Check sheet for the modelled part. Datum: model origin and axes. Units: mm. Face numbers are marked on the shaded views. A direction names the side the tool comes from. Give positions to 0.01 mm unless a question says otherwise; leave off trailing zeros. Order: outer loops, then holes, each group sorted by start corner. A loop starts at its lowest first (then second) coordinate and runs counter-clockwise, first axis right, second up.
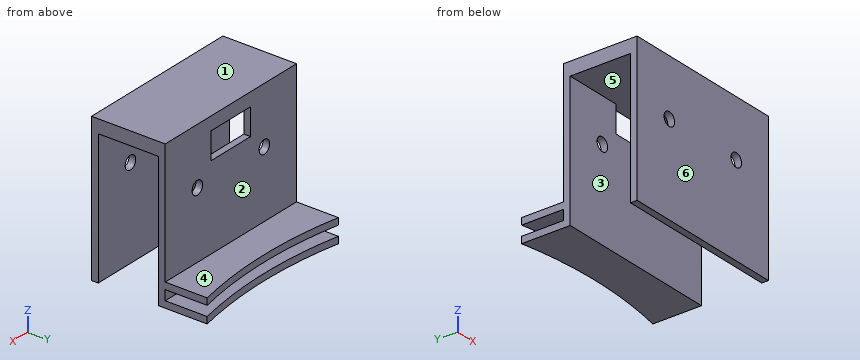
```python
from build123d import *

# Parameters (mm, degrees)
SKETCH_1_W          = 50
SKETCH_1_H          = 44
EXTRUDE_1_DEPTH     = 22
SKETCH_2_W          = 50
SKETCH_2_H          = 2
EXTRUDE_2_DEPTH     = 20
SKETCH_3_W          = 40
SKETCH_3_H          = 18
CUT_EXTRUDE_1_DEPTH = 50
SKETCH_4_R          = 2
CUT_EXTRUDE_2_DEPTH = 22
SKETCH_5_W          = 15
SKETCH_5_H          = 8
CUT_EXTRUDE_3_DEPTH = 2
CUT_EXTRUDE_4_DEPTH = 7


with BuildPart() as part:
    # 스케치1 → 보스-돌출1 (new body)
    with BuildSketch(Plane(origin=(0, 0, 0), x_dir=(1, 0, 0), z_dir=(0, 1, 0))):
        Rectangle(SKETCH_1_W, SKETCH_1_H)
    extrude(amount=EXTRUDE_1_DEPTH)

    # 스케치2 → 보스-돌출2 (add)
    with BuildSketch(Plane(origin=(0, 22, 0), x_dir=(1, 0, 0), z_dir=(0, 1, 0))):
        with Locations((0, 21)):
            Rectangle(SKETCH_2_W, SKETCH_2_H)
        with Locations((0, 16)):
            Rectangle(SKETCH_2_W, SKETCH_2_H)
    extrude(amount=EXTRUDE_2_DEPTH)

    # 스케치3 → 컷-돌출1 (cut)
    with BuildSketch(Plane(origin=(25, 0, 0), x_dir=(0, 0, -1), z_dir=(1, 0, 0))):
        with Locations((2, 11)):
            Rectangle(SKETCH_3_W, SKETCH_3_H)
    extrude(amount=-CUT_EXTRUDE_1_DEPTH, mode=Mode.SUBTRACT)

    # 스케치4 → 컷-돌출2 (cut)
    with BuildSketch(Plane.XZ):
        with Locations((12.75, 5)):
            Circle(SKETCH_4_R)
        with Locations((-12.75, 5)):
            Circle(SKETCH_4_R)
    extrude(amount=-CUT_EXTRUDE_2_DEPTH, mode=Mode.SUBTRACT)

    # 스케치5 → 컷-돌출3 (cut)
    with BuildSketch(Plane(origin=(0, 22, 0), x_dir=(1, 0, 0), z_dir=(0, 1, 0))):
        with Locations((0, -14)):
            Rectangle(SKETCH_5_W, SKETCH_5_H)
    extrude(amount=-CUT_EXTRUDE_3_DEPTH, mode=Mode.SUBTRACT)

    # 스케치7 → 컷-돌출4 (cut)
    with BuildSketch(Plane(origin=(0, 0, -22), x_dir=(-1, 0, 0), z_dir=(0, 0, -1))):
        with BuildLine():
            Line((25, 34.525512861), (25, 42))
            Line((25, 42), (-25, 42))
            Line((-25, 42), (-25, 34.525512861))
            ThreePointArc((-25, 34.525512861), (0, 32), (25, 34.525512861))
        make_face()
    extrude(amount=-CUT_EXTRUDE_4_DEPTH, mode=Mode.SUBTRACT)


solid = part.part
```
Q1. Go/stop test with flat-tipped pins: P1, Ø10, axis at x = 3, y = 29.5, coming from the +Z side; P2, Ø12, axis at x = -19, z = 2.5, coming from the +Y side; P3, Ø2.5, axis at x = 12.75, z = 5, coming from the -Y side. Record where each tip stops, or that it passes through.
Q2. Sectioned sample at C-C, the plane y = 30.5. Record the cut outline in (x, z).
Q3. Material ranges on line 1 (Y direction, x = 6.5, z = 1); line 2 (Z direction, x = 3, y = 21.5); line 3 (Z direction, x = 10, y = 32), recorded low to high.
Q4. Sectioned sample at A-A, the plane z = 5. Record the cut outline in (x, y).
Q5. Sectioned sample at B-B, the plane z = -12.5. Record the cut outline in (x, y).
Q6. Tool access check on the marked faces 1, 2 and 3. Record the directions out of +Z, -Z, +X, -X, +Y, -Y that give a thin tool (end or side, any length) a straight path to the whole face; none if there is none.
Q7. Sectioned sample at D-D, the plane x = 12.75. Record the cut outline in (y, z).
Q8. Draft check along Y on the marked faces 4, 5 and 6. Enter one of: pulls with the +Y half, pulls with the -Y half, needs draft (parallel to the pull), parting line crosses it, or undercut.
Filled in:
1. P1: stops at z = -15
1. P2: stops at y = 22
1. P3: passes through
2. outline: (-25, -22) - (25, -22) - (25, -20) - (-25, -20) - close; (-25, -17) - (25, -17) - (25, -15) - (-25, -15) - close
3. line 1: y = 0 to 2, 20 to 22
3. line 2: z = -22 to 10, 18 to 22
3. line 3: z = -22 to -20, -17 to -15
4. outline: (-25, 0) - (-14.75, 0) - (-14.75, 2) - (-25, 2) - close; (-25, 20) - (-14.75, 20) - (-14.75, 22) - (-25, 22) - close; (-10.75, 0) - (10.75, 0) - (10.75, 2) - (-10.75, 2) - close; (-10.75, 20) - (10.75, 20) - (10.75, 22) - (-10.75, 22) - close; (14.75, 0) - (25, 0) - (25, 2) - (14.75, 2) - close; (14.75, 20) - (25, 20) - (25, 22) - (14.75, 22) - close
5. outline: (-25, 0) - (25, 0) - (25, 2) - (-25, 2) - close; (-25, 20) - (25, 20) - (25, 22) - (-25, 22) - close
6. face 1: +Z, +X, -X, +Y, -Y
6. face 2: +Z, +X, -X, +Y
6. face 3: -Z, +X, -X
7. outline: (0, -22) - (2, -22) - (2, 3) - (0, 3) - close; (0, 7) - (2, 7) - (2, 18) - (20, 18) - (20, 7) - (22, 7) - (22, 22) - (0, 22) - close; (20, -22) - (32.65, -22) - (32.65, -20) - (22, -20) - (22, -17) - (32.65, -17) - (32.65, -15) - (22, -15) - (22, 3) - (20, 3) - close
8. face 4: needs draft
8. face 5: undercut
8. face 6: pulls with the -Y half
